Autodesk Inventor part; units mm, degrees
ref_plane "YZ Plane" through (0, 0, 0) normal (1, 0, 0) x (0, 1, 0)
ref_plane "XZ Plane" through (0, 0, 0) normal (0, 1, 0) x (-1, 0, 0)
ref_plane "XY Plane" through (0, 0, 0) normal (0, 0, 1) x (1, 0, 0)
sketch "スケッチ1" plane through (0, 0, 0) normal (0, 0, 1) x (1, 0, 0)
  line L0 (3, 13.1) -> (-3, 13.1)
  line L1 (-3, 13.1) -> (-3, 17.9)
  line L2 (-3, 17.9) -> (3, 17.9)
  line L3 (3, 17.9) -> (3, 13.1)
  arc A0 (3, 17.6468) -> (-3, 17.6468) centre (0, 0) ccw
  point P0 (0, 13.1)
  dimension "d0" = 17.9
  dimension "d1" = 6
  dimension "d2" = 4.8
extrude "押し出し1" add sketch "スケッチ1" along normal blind 5.5 contours L0 L1 A0 L3
sketch "スケッチ2" plane through (0, 0, 0) normal (0, 0, -1) x (-1, 0, 0)
  line L0 (-2.3, 13.8) -> (2.3, 13.8)
  line L1 (2.3, 13.8) -> (2.3, 17.9)
  line L2 (2.3, 17.9) -> (-2.3, 17.9)
  line L3 (-2.3, 17.9) -> (-2.3, 13.8)
  line L4 (3, 13.1) -> (-3, 13.1)
  line L5 (3, 17.6468) -> (3, 13.1)
  arc A0 (3, 17.6468) -> (-3, 17.6468) centre (0, 0) ccw
  point P0 (0, 13.8)
  point P1 (0, 13.1)
  point P2 (2.3, 17.7516)
  point P3 (-2.3, 17.7516)
  dimension "d5" = 0.7
  dimension "d6" = 0.7
extrude "押し出し2" cut sketch "スケッチ2" against normal blind 3.6 contours L3 A0 L1 L0
fillet "フィレット1" radius 0.2 4 edges at (3, 13.1, 2.75) (2.3, 13.8, 1.8) (-2.3, 13.8, 1.8) (-3, 13.1, 2.75)
properties part number "555_CapAccessory" material "アセタール樹脂、白"
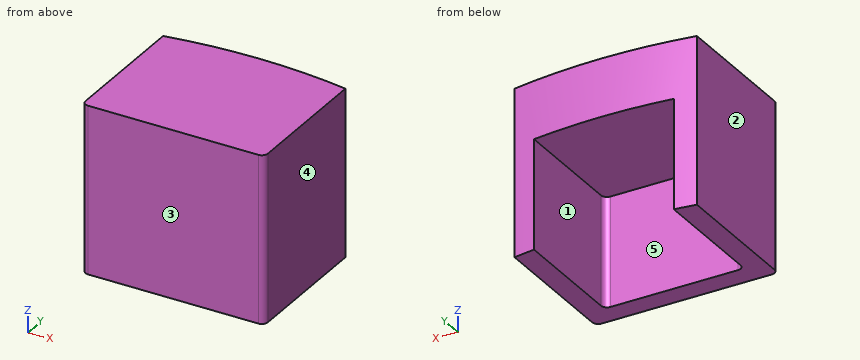
The model under review builds one solid part; all positions refer to its coordinate system, in mm. Face numbers are marked on the shaded views. A direction names the side the tool comes from. Give positions to 0.01 mm unless a question says otherwise; leave off trailing zeros. Order: outer loops, then holes, each group sorted by start corner. A loop starts at its lowest first (then second) coordinate and runs counter-clockwise, first axis right, second up. Notation, with made-up numbers: (-5.5, 57) -> (18.5, 57) arc R15 ccw to (18.5, 80) -> close; hole circle Ø1 at (44, 40.25). An arc over 180 degrees is marked (long way). Write item = value, one per line. Start each with the question number.
(1) Tool access review of the marked faces 4 and 5: name each direction out of +Z, -Z, +X, -X, +Y, -Y from which nothing blocks a thin tool from reaching the whole face with its end or side.
(2) Take a section at D-D (z = 4.85). Write out the cut boundary in (x, y), plus the area to 3 significant figures.
(3) For pin 1 Ø1 at (x, z) = (-1, 5) entering from +Y, flat-tipped, find the tip position at first contact; note if it passes through.
(4) Take a section at A-A (y = 16.5). Write out the cut boundary in (x, z).
(5) Draft analysis for pull direction X (two halves, no side actions). For the marked faces 1, 2 and 3, state which applies: +X half, -X half, draft (parallel to the pull), parting line (faces both ways), or undercut.
(6) For L1, parallel to X at y = 16.05, z = 0.6; L2, parallel to Y at x = 2.1, z = 2.6; L3, parallel to Z at x = -0.7, y = 14.8, list the stretches that pass through material, from the lowest coordinate up. Write a range as from..to.
(7) Take a section at B-B (z = 2). Write out the cut boundary in (x, y).
(8) Take a section at C-C (x = 0.9). Write out the cut boundary in (y, z).
Returned:
q1.face_4 = +Z, -Z, +X, +Y, -Y
q1.face_5 = -Z, +Y
q2.outline = (-3, 13.3) arc R0.2 ccw to (-2.8, 13.1) -> (2.8, 13.1) arc R0.2 ccw to (3, 13.3) -> (3, 17.65) arc R17.9 ccw to (-3, 17.65) -> close
q2.area = 28.3 mm²
q3.pin_1 = 17.89
q4.outline = (-3, 0) -> (-2.3, 0) -> (-2.3, 3.6) -> (2.3, 3.6) -> (2.3, 0) -> (3, 0) -> (3, 5.5) -> (-3, 5.5) -> close
q5.face_1 = undercut
q5.face_2 = -X half
q5.face_3 = draft
q6.L1 = -3..-2.3, 2.3..3
q6.L2 = 13.1..13.8
q6.L3 = 3.6..5.5
q7.outline = (-3, 13.3) arc R0.2 ccw to (-2.8, 13.1) -> (2.8, 13.1) arc R0.2 ccw to (3, 13.3) -> (3, 17.65) arc R17.9 ccw to (2.3, 17.75) -> (2.3, 14) arc R0.2 cw to (2.1, 13.8) -> (-2.1, 13.8) arc R0.2 cw to (-2.3, 14) -> (-2.3, 17.75) arc R17.9 ccw to (-3, 17.65) -> close
q8.outline = (13.1, 0) -> (13.8, 0) -> (13.8, 3.6) -> (17.88, 3.6) -> (17.88, 5.5) -> (13.1, 5.5) -> close
